Read the model definition and answer for the solid it produces. Units are mm, in the model's axes. A direction names the side the tool comes from. Give positions to 0.01 mm unless a question says otherwise; leave off trailing zeros. Write each loop counter-clockwise with the first axis right and the second up, starting at its lowest first coordinate (ties: lowest second). Pieces come first, ordered by that corner, then holes. Notation, with made-up numbers: (-18.75, -37.75) - (26.25, -37.75) arc R25 cw to (26.25, -17.75) - close; hole circle Ø9 at (26.5, 7.5). An arc over 180 degrees is marked (long way). Answer as a JSON object with one key per item and string values. Group by question number.
```python
from build123d import *
from build123d import SkipClean  # not in build123d's __all__

# Parameters (mm, degrees)
F0_R      = 12.5377374601
F1_DEPTH  = 6.21636
F3_DEPTH  = 43.11412
F5_DEPTH  = 2.29052
F6_R      = 9.2054650922
F7_DEPTH  = 4.2521
F8_R      = 8.8363001854
F9_DEPTH  = 13.21401
F10_R     = 3.2055120306
F11_DEPTH = 28.79148
F12_R     = 5.1967625573
F13_DEPTH = 1.68604
F14_R     = 3.2868447942
F15_DEPTH = 33.07979
F16_R     = 6.7713245086
F17_DEPTH = 3.883
F20_DEPTH = 42.80702
F22_DEPTH = 12.5


# Not quite as in the source:
# - a fillet or chamfer that OpenCascade refuses, or shapes differently, is made with other operations: its cross-section is extruded or revolved along the edge and cut away or added
# - after a boolean that leaves OpenCascade's solid faulty, fix() repairs it


with BuildPart() as f1:
    # F0 (on Front) → F1 (new body, symmetric)
    with BuildSketch(Plane.XZ):
        Circle(F0_R)
    extrude(amount=F1_DEPTH, both=True)

    # F2 (on face) → F3 (cut)
    with BuildSketch(Plane.XZ.offset(6.21636)):
        Polygon((-1.5670347233, 8.3723281259), (-8.0341662075, 2.8290721839), (-6.4671314842, -5.5432559419), (1.5670347233, -8.3723281259), (8.0341662075, -2.8290721839), (6.4671314842, 5.5432559419), align=None)
    extrude(amount=-F3_DEPTH, mode=Mode.SUBTRACT)

    # F4 (on Front) → F5 (join, symmetric)
    with BuildSketch(Plane.XZ):
        with BuildLine():
            ThreePointArc((-32.5207371804, -47.4863935268), (-30.3092801317, -44.4938571079), (-29.5258178112, -40.8562750417))
            ThreePointArc((-29.5258178112, -40.8562750417), (-35.5217487699, -32.4889275753), (-45.3723830373, -35.4770199791))
            ThreePointArc((-45.3723830373, -35.4770199791), (-44.3951798921, -47.3124631688), (-32.5207371804, -47.4863935268))
        make_face()
        with BuildLine():
            ThreePointArc((-45.3723830373, -35.4770199791), (-35.5217487699, -32.4889275753), (-29.5258178112, -40.8562750417))
            ThreePointArc((-29.5258178112, -40.8562750417), (-30.3092801317, -44.4938571079), (-32.5207371804, -47.4863935268))
            Line((-32.5207371804, -47.4863935268), (-12.0985076262, -29.4936502279))
            ThreePointArc((-12.0985076262, -29.4936502279), (0, -24.9242672402), (12.0985076262, -29.4936502279))
            Line((12.0985076262, -29.4936502279), (32.5207371804, -47.4863935268))
            ThreePointArc((32.5207371804, -47.4863935268), (32.3290561012, -34.4000869145), (45.3723830373, -35.4770199791))
            Line((45.3723830373, -35.4770199791), (12.0060265403, 8.0061388902))
            ThreePointArc((12.0060265403, 8.0061388902), (0, 13.9267959918), (-12.0060265403, 8.0061388902))
            Line((-12.0060265403, 8.0061388902), (-45.3723830373, -35.4770199791))
        make_face()
        with BuildLine():
            ThreePointArc((47.1984181821, -40.8562750417), (46.729465463, -38.0159058149), (45.3723830373, -35.4770199791))
            ThreePointArc((45.3723830373, -35.4770199791), (32.3290561012, -34.4000869145), (32.5207371804, -47.4863935268))
            ThreePointArc((32.5207371804, -47.4863935268), (41.9997000629, -48.9091129066), (47.1984181821, -40.8562750417))
        make_face()
    extrude(amount=F5_DEPTH, both=True)

    # F6 (on face) → F7 (join, symmetric)
    with BuildSketch(Plane.XZ.offset(2.29052)):
        with Locations((-38.3621179966, -40.8562750417)):
            Circle(F6_R)
    extrude(amount=F7_DEPTH, both=True)

    # F8 (on face) → F9 (join)
    with BuildSketch(Plane.XZ.offset(2.29052)):
        with Locations((38.3621179966, -40.8562750417)):
            Circle(F8_R)
    with SkipClean():  # cleaning this boolean's faces spoils the solid; the shape is the same uncleaned
        extrude(amount=F9_DEPTH)

    # F10 (on face) → F11 (cut)
    with BuildSketch(Plane.XZ.offset(6.54262)):
        with Locations((-38.3621179966, -40.8562750417)):
            Circle(F10_R)
    extrude(amount=-F11_DEPTH, mode=Mode.SUBTRACT)

    add(f1.part.fix(), mode=Mode.REPLACE)

    # F12 (on face) → F13 (cut)
    with BuildSketch(Plane.XZ.offset(6.54262)):
        with Locations((-38.3621179966, -40.8562750417)):
            Circle(F12_R)
    extrude(amount=-F13_DEPTH, mode=Mode.SUBTRACT)

    # F14 (on face) → F15 (cut)
    with BuildSketch(Plane.XZ.offset(15.50453)):
        with Locations((38.3621179966, -40.8562750417)):
            Circle(F14_R)
    extrude(amount=-F15_DEPTH, mode=Mode.SUBTRACT)

    # F16 (on face) → F17 (cut)
    with BuildSketch(Plane.XZ.offset(15.50453)):
        with Locations((38.3621179966, -40.8562750417)):
            Circle(F16_R)
    extrude(amount=-F17_DEPTH, mode=Mode.SUBTRACT)

    # F18: chamfer of 2.54 on 1 edges, made by hand

    # F18_s1 → F18_t2 (revolve, cut)
    with BuildSketch(Plane.XY.offset(-40.8562750417)):
        Polygon((47.1984181821, -12.96453), (44.6584181821, -15.50453), (47.1984181821, -15.50453), align=None)
    revolve(axis=Axis((38.3621179966, -15.50453, -40.8562750417), (0, -1, 0)), mode=Mode.SUBTRACT)

    # F19 (on face) → F20 (cut)
    with BuildSketch(Plane.XZ.offset(2.29052)):
        Polygon((7.5046534745, -4.3328137037), (7.5046534745, 4.3328137037), (0, 8.6656274074), (-7.5046534745, 4.3328137037), (-7.5046534745, -4.3328137037), (0, -8.6656274074), align=None)
    extrude(amount=-F20_DEPTH, mode=Mode.SUBTRACT)

    # F21 (on Front) → F22 (cut, symmetric)
    with BuildSketch(Plane.XZ):
        Polygon((8.97537597, 4.8977579377), (0.2461051893, 10.2217825674), (-8.7292707806, 5.3240246297), (-8.97537597, -4.8977579377), (-0.2461051893, -10.2217825674), (8.7292707806, -5.3240246297), align=None)
    extrude(amount=F22_DEPTH, both=True, mode=Mode.SUBTRACT)


solid = f1.part
```
1) Find section A-A, the plane y = 3.75. Write down the section's boundary in (x, z), and give its area (3 significant figures).
2) Find section B-B, the plane x = 4. Write down the section's boundary in (y, z), and give its area (3 significant figures).
3) Which of the six approach directions +Z, -Z, +X, -X, +Y, -Y give full straight-line access (tool end or side, diameter ignored) to faces 1 (the flat face through (-4.672, -0.087, -7.523)), 2 (the cylindrical face through (-44.527, 2.124, -47.187)), 3 (the flat face through (0, -2.291, -23))?
4) Find section C-C, the plane y = -0.5. Write down the section's boundary in (x, z).
5) Flat-ended cylindrical pins translate along their axes: pin 1 Ø16.5 at (x, z) = (-38.36, -40.86) entering from +Y; pin 2 Ø10.5 at (x, z) = (-38.36, -40.86) entering from -Y; pin 3 Ø12 at (x, y) = (33.5, -2.5) entering from -Z; pin 4 Ø4 at (x, z) = (31.5, -42) entering from -Y. Find the tip coordinate at first contact, or state that the pin passes through.
6) For a pull along X with two mould halves and no side action, classify faces 4 (the flat face through (-0.7, 2.291, -24.5)), 5 (the flat face through (35, -11.622, -42)), 6 (the cylindrical face through (11.959, 4.226, 3.766)) as released by +X, released by -X, zero draft, split by the parting line, or undercut.
7) Find the intervals of material crossed by line 1 (Z direction, x = -41.5, y = -5); line 2 (Y direction, x = -43, z = -34); line 3 (Z direction, x = 37, y = -12.5), in increasing order. Write a range as [from, to].
8) Find section D-D, the plane z = 0. Write down the section's boundary in (x, y), and give its area (3 significant figures).
Values follow:
{
 "1": {"outline": "circle Ø25.08 at (0, 0); hole (-8.98, -4.9) - (-0.25, -10.22) - (8.73, -5.32) - (8.98, 4.9) - (0.25, 10.22) - (-8.73, 5.32) - close", "area": "222 mm2"},
 "2": {"outline": "(-6.22, -11.88) - (-2.29, -11.88) - (-2.29, -25.37) - (2.29, -25.37) - (2.29, -11.88) - (6.22, -11.88) - (6.22, -7.9) - (-6.22, -7.9) - close; (-6.22, 7.93) - (6.22, 7.93) - (6.22, 11.88) - (2.29, 11.88) - (2.29, 13.39) - (-2.29, 13.39) - (-2.29, 11.88) - (-6.22, 11.88) - close", "area": "167 mm2"},
 "3": {"face 1": "+Y, -Y", "face 2": "+Y", "face 3": "-Y"},
 "4": {"outline": "(-43.8, -33.43) arc R9.21 ccw (long way) to (-30.58, -45.78) - (-12.1, -29.49) arc R18.3 cw to (12.1, -29.49) - (32.52, -47.49) arc R8.84 ccw to (45.37, -35.48) - (12.01, 8.01) arc R15.13 ccw to (-12.01, 8.01) - close; hole circle Ø6.41 at (-38.36, -40.86); hole (-8.98, -4.9) - (-0.25, -10.22) - (8.73, -5.32) - (8.98, 4.9) - (0.25, 10.22) - (-8.73, 5.32) - close; hole circle Ø6.57 at (38.36, -40.86)"},
 "5": {"pin 1": "stops at y = 2.29", "pin 2": "stops at y = -6.54", "pin 3": "stops at z = -49.69", "pin 4": "stops at y = -15.03"},
 "6": {"face 4": "zero draft", "face 5": "undercut", "face 6": "split by the parting line"},
 "7": {"line 1": "z = [-49.51, -45], [-36.71, -32.2]", "line 2": "y = [-6.54, 2.29]", "line 3": "z = [-49.59, -47.49], [-34.22, -32.13]"},
 "8": {"outline": "(-18.15, -2.29) - (-12.54, -2.29) - (-12.54, -6.22) - (-8.86, -6.22) - (-8.86, 6.22) - (-12.54, 6.22) - (-12.54, 2.29) - (-18.15, 2.29) - close; (8.86, -6.22) - (12.54, -6.22) - (12.54, -2.29) - (18.15, -2.29) - (18.15, 2.29) - (12.54, 2.29) - (12.54, 6.22) - (8.86, 6.22) - close", "area": "143 mm2"}
}
